from build123d import *

# Parameters (mm, degrees)
SKETCH1_W           = 16.8
SKETCH1_H           = 13.8
BOSS_EXTRUDE1_DEPTH = 6
CUT_EXTRUDE1_REACH  = 14.417
SKETCH2_R           = 6.1
FILLET1_R           = 2


with BuildPart() as part:
    # Sketch1 → Boss-Extrude1 (new body)
    with BuildSketch(Plane.XY):
        Rectangle(SKETCH1_W, SKETCH1_H)
    extrude(amount=BOSS_EXTRUDE1_DEPTH)

    # Sketch2 → Cut-Extrude1 (cut, up to next)
    with BuildSketch(Plane.XY.offset(6), mode=Mode.PRIVATE) as cut_extrude1_sk1:
        Circle(SKETCH2_R)
    cut_extrude1_tool1 = extrude(cut_extrude1_sk1.sketch, amount=-CUT_EXTRUDE1_REACH, mode=Mode.PRIVATE) & part.part
    add(cut_extrude1_tool1.solids().sort_by_distance((0, 0, 6))[0], mode=Mode.SUBTRACT)

    # Fillet1
    fillet1_edges = [part.edges().sort_by_distance(p)[0] for p in [
        (8.4, -6.9, 3),
        (-8.4, -6.9, 3),
        (-8.4, 6.9, 3),
        (8.4, 6.9, 3),
    ]]
    fillet(fillet1_edges, radius=FILLET1_R)


solid = part.part
Could you check a few things on this model? Use its own coordinates, in mm. Coordinates: 2 decimals unless noted, no trailing zeros. Order: outer loops, then holes, each group sorted by start corner. A loop starts at its lowest first (then second) coordinate and runs counter-clockwise, first axis right, second up.
Q1. Suppose I cut it at A-A on z = 3.1. Please give me the cut outline in (x, y), and give its area (3 significant figures).
Q2. Suppose I cut it at D-D on x = -7.5. Please give me the cut outline in (y, z).
Q3. Suppose I cut it at C-C on y = 0. Please give me the cut outline in (x, z), and give its area (3 significant figures).
Q4. Suppose I cut it at B-B on x = 0. Please give me the cut outline in (y, z).
Q5. Will this pin go through, and if not, where does the flat tip stop? pin 1 (7.5 mm diameter, centred on x = 0, y = 0, fed in from +Z).
Q6. Please list where these lines run through material, in increasing order: L1, parallel to Y at x = 0, z = 4.05; L2, parallel to Y at x = 2.75, z = 3; L3, parallel to X at y = 0.75, z = 4.35.
Q7. Thinking about a two-plate mould opening in X: for faces 1 (the flat face through (0, 6.9, 3)), 2 (the flat face through (-8.4, 0, 3)), 3 (the cylindrical face through (-6.094, 0.268, 3.042)), which applies, released by +X, released by -X, zero draft, split by the parting line, or undercut?
Answer:
1. outline: (-8.4, -4.9) arc R2 ccw to (-6.4, -6.9) - (6.4, -6.9) arc R2 ccw to (8.4, -4.9) - (8.4, 4.9) arc R2 ccw to (6.4, 6.9) - (-6.4, 6.9) arc R2 ccw to (-8.4, 4.9) - close; hole circle Ø12.2 at (0, 0)
1. area: 112 mm2
2. outline: (-6.57, 0) - (6.57, 0) - (6.57, 6) - (-6.57, 6) - close
3. outline: (-8.4, 0) - (-6.1, 0) - (-6.1, 6) - (-8.4, 6) - close; (6.1, 0) - (8.4, 0) - (8.4, 6) - (6.1, 6) - close
3. area: 27.6 mm2
4. outline: (-6.9, 0) - (-6.1, 0) - (-6.1, 6) - (-6.9, 6) - close; (6.1, 0) - (6.9, 0) - (6.9, 6) - (6.1, 6) - close
5. pin 1: passes through
6. L1: y = -6.9 to -6.1, 6.1 to 6.9
6. L2: y = -6.9 to -5.44, 5.44 to 6.9
6. L3: x = -8.4 to -6.05, 6.05 to 8.4
7. face 1: zero draft
7. face 2: released by -X
7. face 3: undercut
